```python
from build123d import *

# Parameters (mm, degrees)
PROFILE_SKETCH_R              = 10
PROFILE_SKETCH_R_2            = 5
CYLINDER_EXTRUDE_DEPTH        = 12
LIP_RING_SKETCH_R             = 7
LIP_RING_SKETCH_R_2           = 5
BOTTOM_LIP_RING_EXTRUDE_DEPTH = 1
BOTTOM_RING_FILLET_R          = 1
TOP_START                     = -13
SKETCH2_2_R                   = 7
SKETCH2_2_R_2                 = 5
TOP_LIP_RING_EXTRUDE_DEPTH    = 1
TOP_RING_FILLET_R             = 1


with BuildPart() as part:
    # Profile Sketch → Cylinder Extrude (new body)
    with BuildSketch(Plane(origin=(0, 0, 0), x_dir=(1, 0, 0), z_dir=(0, 1, 0))):
        with Locations(Location((0, 0, 0), (0, 0, 270))):
            Circle(PROFILE_SKETCH_R)
        with Locations(Location((0, 0, 0), (0, 0, 270))):
            Circle(PROFILE_SKETCH_R_2, mode=Mode.SUBTRACT)
    extrude(amount=CYLINDER_EXTRUDE_DEPTH)

    # Lip Ring Sketch → Bottom Lip Ring Extrude (add)
    with BuildSketch(Plane(origin=(0, 12, 0), x_dir=(1, 0, 0), z_dir=(0, 1, 0))):
        with Locations(Location((0, 0, 0), (0, 0, 270))):
            Circle(LIP_RING_SKETCH_R)
        with Locations(Location((0, 0, 0), (0, 0, 270))):
            Circle(LIP_RING_SKETCH_R_2, mode=Mode.SUBTRACT)
    extrude(amount=BOTTOM_LIP_RING_EXTRUDE_DEPTH)

    # Bottom Ring Fillet
    bottom_ring_fillet_edges = [part.edges().sort_by_distance(p)[0] for p in [
        (0, 13, -7),
        (0, 13, -5),
    ]]
    fillet(bottom_ring_fillet_edges, radius=BOTTOM_RING_FILLET_R - 0.0001)  # a hair under: the kernel refuses the full size

    # Sketch2<2> → Top Lip Ring Extrude (add)
    with BuildSketch(Plane(origin=(0, 12, 0), x_dir=(1, 0, 0), z_dir=(0, 1, 0)).offset(TOP_START)):
        with Locations(Location((0, 0, 0), (0, 0, 270))):
            Circle(SKETCH2_2_R)
        with Locations(Location((0, 0, 0), (0, 0, 270))):
            Circle(SKETCH2_2_R_2, mode=Mode.SUBTRACT)
    extrude(amount=TOP_LIP_RING_EXTRUDE_DEPTH)

    # Top Ring Fillet
    top_ring_fillet_edges = [part.edges().sort_by_distance(p)[0] for p in [
        (0, -1, -7),
        (0, -1, -5),
    ]]
    fillet(top_ring_fillet_edges, radius=TOP_RING_FILLET_R - 0.0001)  # a hair under: the kernel refuses the full size


solid = part.part
```
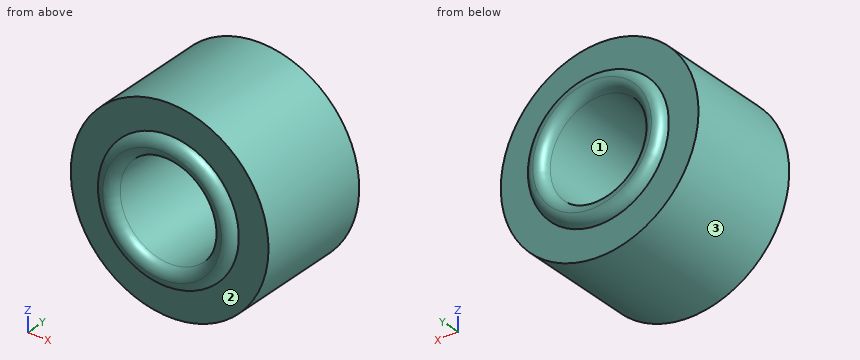
Input: part model. Units: mm. Frame: model coordinates. Face numbers are marked on the shaded views. Round coordinates to 2 decimals unless told otherwise and drop trailing zeros. Loops run counter-clockwise (first coordinate to the right, second up) from the corner with the lowest first, then second, coordinate; pieces in that order, holes last. Notation, with made-up numbers: (4.25, 43.5) -> (20.25, 43.5) arc R25 cw to (20.25, 69.5) -> close; hole circle Ø2 at (-33.5, 60.5). An arc over 180 degrees is marked (long way). Use one line per item in the form item = value. Start each with the question number.
Item 1: Contact query for flat-ended pins moving along their axis: pin 1 Ø2 at (x, z) = (7, -4.5) entering from -Y; pin 2 Ø2 at (y, z) = (3, 5.5) entering from -X; pin 3 Ø5 at (x, y) = (-3.5, 5) entering from -Z. Output: stop coordinate, or through.
Item 2: Section query B-B on y = 6.5. Return the cut outline in (x, z).
Item 3: Material intervals for L1, parallel to X at y = 3.5, z = 0; L2, parallel to Y at x = -4.5, z = 6.5; L3, parallel to X at y = 3.5, z = -4.5, sorted ascending. Write a range as from..to.
Item 4: Mould query, pull axis X, two halves, no side actions, for the marked faces 1, 2 and 3. Classes: pulls with the +X half, pulls with the -X half, needs draft (parallel to the pull), parting line crosses it, or undercut.
Ans:
q1.pin_1 = 0
q1.pin_2 = -8.93
q1.pin_3 = -9.95
q2.outline = circle Ø20 at (0, 0); hole circle Ø10 at (0, 0)
q3.L1 = -10..-5, 5..10
q3.L2 = 0..12
q3.L3 = -8.93..-2.18, 2.18..8.93
q4.face_1 = undercut
q4.face_2 = needs draft
q4.face_3 = parting line crosses it
